Check sheet for the modelled part. Datum: model origin and axes. Units: mm. A direction names the side the tool comes from. Round coordinates to 2 decimals unless told otherwise and drop trailing zeros. Order: outer loops, then holes, each group sorted by start corner. A loop starts at its lowest first (then second) coordinate and runs counter-clockwise, first axis right, second up. Notation, with made-up numbers: M 27.5,-26.5 L 54.5,-26.5 A11 cw 54.5,-18.5 Z; hole C 21,-4 d6. An arc over 180 degrees is marked long. One line per item, written item: value. Start each with the question number.
(1) Depth check by flat-ended pin: pin 1 Ø8.5 at (x, z) = (-3, -13.5) entering from +Y; pin 2 Ø10 at (x, y) = (-4, -2) entering from -Z; pin 3 Ø4 at (y, z) = (-53.5, -40) entering from -X; pin 4 Ø5 at (x, y) = (-7, -38) entering from -Z. Enter the tip coordinate at first touch or a pass-through.
(2) Access from +Z, -Z, +X, -X, +Y, -Y to the whole of each face (thin tool, end or side, straight path). Record for faces 1 (the face through (0.27, -1.22, 1.23)), 2 (the face through (-5, -24.1, -13.4)), 3 (the face through (0, -5, -29.7)), 4 (the face through (0, -2, 0)), 5 (the face through (7.686, 1.075, 1.232)).
(3) Cross-section at D-D, the plane x = 6. Enter the section's corners in (y, z).
(4) Thickness scan on L1, parallel to Y at x = 0, z = 1.55; L2, parallel to Z at x = -4.5, y = -14.5; L3, parallel to Y at x = 0, z = -27.75. Record the ranges inside material, lowest first.
(5) Release check for a two-part mould opening along Y. For faces 6 (the face through (0, -72, -22)), 7 (the face through (0, 10, -28)), 8 (the face through (0, -8, 1)) record: released by +Y, released by -Y, zero draft, split by the parting line, or undercut.
(6) Cross-section at A-A, the plane y = 6. Enter the section's corners in (x, z), and give its area (3 significant figures).
(7) Cross-section at B-B, the plane x = 0. Count the separate pieces of the cut face and the enclosed holes in it, and give its area (3 significant figures).
from build123d import *

# Parameters (mm, degrees)
SKETCH2_R           = 10
BOSS_EXTRUDE1_DEPTH = 2.5
SKETCH4_R           = 1.25
CUT_EXTRUDE3_DEPTH  = 10
SKETCH5_R           = 2
CUT_EXTRUDE4_DEPTH  = 10
CIRPATTERN1_COUNT   = 4
BOSS_EXTRUDE2_START = -2.5
BOSS_EXTRUDE2_DEPTH = 2.5
SKETCH8_W           = 20
SKETCH8_H           = 2.5
BOSS_EXTRUDE3_DEPTH = 27.2
BOSS_EXTRUDE4_START = 2.5
SKETCH10_R          = 2
BOSS_EXTRUDE4_DEPTH = 2.5
FILLET1_R           = 5
SKETCH12_W          = 6
SKETCH12_H          = 32.2
BOSS_EXTRUDE5_DEPTH = 50
SKETCH13_W          = 6
SKETCH13_H          = 50
BOSS_EXTRUDE6_DEPTH = 18
FILLET2_R           = 7
FILLET3_R           = 15


with BuildPart() as part:
    # Sketch2 → Boss-Extrude1 (new body)
    with BuildSketch(Plane(origin=(0, 0, 0), x_dir=(-1, 0, 0), z_dir=(0, 0, -1))):
        Circle(SKETCH2_R)
    extrude(amount=-BOSS_EXTRUDE1_DEPTH)

    # Sketch4 → Cut-Extrude3 (cut)
    with BuildSketch(Plane(origin=(0, 0, 0), x_dir=(-1, 0, 0), z_dir=(0, 0, -1))):
        Circle(SKETCH4_R)
    extrude(amount=-CUT_EXTRUDE3_DEPTH, mode=Mode.SUBTRACT)

    # Sketch5 → Cut-Extrude4 (cut)
    with BuildSketch(Plane(origin=(0, 0, 0), x_dir=(-1, 0, 0), z_dir=(0, 0, -1))):
        with Locations((0, 6)):
            Circle(SKETCH5_R)
    cut_extrude4 = extrude(amount=-CUT_EXTRUDE4_DEPTH, mode=Mode.SUBTRACT)

    # CirPattern1: Cut-Extrude4 ×4 about axis
    cirpattern1_axis = Axis((0, 0, 0), (0, 0, 1))
    for i in range(1, CIRPATTERN1_COUNT):
        add(cut_extrude4.rotate(cirpattern1_axis, i * 360 / CIRPATTERN1_COUNT), mode=Mode.SUBTRACT)

    # Sketch6 → Boss-Extrude2 (add)
    with BuildSketch(Plane.XY.offset(2.5).offset(BOSS_EXTRUDE2_START)):
        with BuildLine():
            Line((-10, 0), (-10, -22))
            Line((-10, -22), (10, -22))
            Line((10, -22), (10, 0))
            ThreePointArc((10, 0), (0, -10), (-10, 0))
        make_face()
    extrude(amount=BOSS_EXTRUDE2_DEPTH)

    # Sketch8 → Boss-Extrude3 (add)
    with BuildSketch(Plane(origin=(0, 0, 0), x_dir=(-1, 0, 0), z_dir=(0, 0, -1))):
        with Locations((0, -20.75)):
            Rectangle(SKETCH8_W, SKETCH8_H)
    extrude(amount=BOSS_EXTRUDE3_DEPTH)

    # Sketch10 → Boss-Extrude4 (add)
    with BuildSketch(Plane(origin=(0, 0, -27.2), x_dir=(-1, 0, 0), z_dir=(0, 0, -1)).offset(BOSS_EXTRUDE4_START)):
        with BuildLine():
            Line((-10, -22), (10, -22))
            Line((10, -22), (10, 0))
            ThreePointArc((10, 0), (0, 10), (-10, 0))
            Line((-10, 0), (-10, -22))
        make_face()
        Circle(SKETCH10_R, mode=Mode.SUBTRACT)
    extrude(amount=-BOSS_EXTRUDE4_DEPTH)

    # Fillet1
    fillet1_edges = [part.edges().sort_by_distance(p)[0] for p in [
        (0, -19.5, 0),
        (0, -19.5, -27.2),
    ]]
    fillet(fillet1_edges, radius=FILLET1_R)

    # Sketch12 → Boss-Extrude5 (add)
    with BuildSketch(Plane.XZ.offset(22)):
        with Locations((0, -13.6)):
            Rectangle(SKETCH12_W, SKETCH12_H)
    extrude(amount=BOSS_EXTRUDE5_DEPTH)

    # Sketch13 → Boss-Extrude6 (add)
    with BuildSketch(Plane(origin=(0, 0, -29.7), x_dir=(-1, 0, 0), z_dir=(0, 0, -1))):
        with Locations((0, -47)):
            Rectangle(SKETCH13_W, SKETCH13_H)
    extrude(amount=BOSS_EXTRUDE6_DEPTH)

    # Fillet2
    fillet2_edges = [part.edges().sort_by_distance(p)[0] for p in [
        (-3, -22, -13.6),
        (3, -22, -13.6),
    ]]
    fillet(fillet2_edges, radius=FILLET2_R - 0.0001)  # a hair under: the kernel refuses the full size

    # Fillet3
    fillet3_edges = [part.edges().sort_by_distance(p)[0] for p in [
        (0, -22, -29.7),
    ]]
    fillet(fillet3_edges, radius=FILLET3_R)


solid = part.part
Values found:
1. pin 1: y = -19.5
1. pin 2: z = -29.7
1. pin 3: x = -3
1. pin 4: through
2. face 1: +Z, -Z
2. face 2: +Z, -Z, -X, -Y
2. face 3: -Z, +Y
2. face 4: +X, -X, +Y
2. face 5: +Z
3. outline: M -23.26,-29.7 L 8,-29.7 L 8,-27.2 L -14.5,-27.2 A5 cw -19.5,-22.2 L -19.5,-5 A5 cw -14.5,0 L -2,0 L -2,2.5 L -23.26,2.5 Z; M 2,0 L 8,0 L 8,2.5 L 2,2.5 Z
4. L1: -72 to -8, -4 to -1.25, 1.25 to 4, 8 to 10
4. L2: -29.7 to -27.2, 0 to 2.5
4. L3: -72 to -2, 2 to 10
5. face 6: released by -Y
5. face 7: released by +Y
5. face 8: undercut
6. outline: M -8,-29.7 L 8,-29.7 L 8,-27.2 L -8,-27.2 Z; M -8,0 L -2,0 L -2,2.5 L -8,2.5 Z; M 2,0 L 8,0 L 8,2.5 L 2,2.5 Z
6. area: 70.0 mm^2
7. separate pieces: 5
7. enclosed holes: 0
7. area: 2,760 mm^2
